Geometry check sheet. Reference: the model listing, model coordinates, mm. A direction names the side the tool comes from. Coordinates: 2 decimals unless noted, no trailing zeros. Loops run counter-clockwise (first coordinate to the right, second up) from the corner with the lowest first, then second, coordinate; pieces in that order, holes last. Notation, with made-up numbers: (45.25, 0.5) -> (62.25, 0.5) arc R15 cw to (62.25, 7.5) -> close; hole circle Ø11 at (57, 48.25). An arc over 180 degrees is marked (long way). Answer as a JSON object with one key per item and string values.
from build123d import *

# Parameters (mm, degrees)
ESQUISSE1_W             = 33.4
ESQUISSE1_H             = 33.4
BOSS_EXTRU_1_DEPTH      = 7
ESQUISSE2_R             = 8.175
ENL_V_MAT_EXTRU_1_DEPTH = 3
ESQUISSE3_W             = 39.4
ESQUISSE3_H             = 39.4
BOSS_EXTRU_2_DEPTH      = 2
BOSS_EXTRU_3_DEPTH      = 10
CONG_1_R                = 2


with BuildPart() as part:
    # Esquisse1 → Boss.-Extru.1 (new body)
    with BuildSketch(Plane.XY):
        Rectangle(ESQUISSE1_W, ESQUISSE1_H)
    extrude(amount=BOSS_EXTRU_1_DEPTH)

    # Esquisse2 → Enlèv. mat.-Extru.1 (cut)
    with BuildSketch(Plane.XY.offset(7)):
        with Locations((0, -2.7)):
            Circle(ESQUISSE2_R)
    extrude(amount=-ENL_V_MAT_EXTRU_1_DEPTH, mode=Mode.SUBTRACT)

    # Esquisse3 → Boss.-Extru.2 (add)
    with BuildSketch(Plane(origin=(0, 0, 0), x_dir=(-1, 0, 0), z_dir=(0, 0, -1))):
        Rectangle(ESQUISSE3_W, ESQUISSE3_H)
    extrude(amount=BOSS_EXTRU_2_DEPTH)

    # Esquisse4 → Boss.-Extru.3 (add)
    with BuildSketch(Plane(origin=(0, 0, -2), x_dir=(-1, 0, 0), z_dir=(0, 0, -1))):
        Polygon((19.7, 19.7), (-19.7, 19.7), (-19.7, -19.7), (-16.7, -19.7), (-16.7, 16.7), (19.7, 16.7), align=None)
    extrude(amount=BOSS_EXTRU_3_DEPTH)

    # Congé1
    cong_1_edges = [part.edges().sort_by_distance(p)[0] for p in [
        (19.7, 19.7, -6),
        (-16.7, 16.7, 3.5),
        (16.7, 16.7, 3.5),
        (16.7, -16.7, 3.5),
        (-16.7, -16.7, 3.5),
    ]]
    fillet(cong_1_edges, radius=CONG_1_R)


solid = part.part
1. Tool access check on faces 1 (the face through (0, -3, 4)), 2 (the face through (-16.1, -16.13, 3.55)), 3 (the face through (0, -16.7, 3)). Record the directions out of +Z, -Z, +X, -X, +Y, -Y that give a thin tool (end or side, any length) a straight path to the whole face; none if there is none.
Evaluation:
{"face 1": "+Z", "face 2": "+Z, -X, -Y", "face 3": "+Z, +X, -X, -Y"}
2. Section check A-A, the plane y = -2.7. Record the boundary of the cut face in (x, z) (3 decimals), then the cut area to 3 significant figures.
Evaluation:
{"outline": "(-19.7, -2) -> (16.7, -2) -> (16.7, -12) -> (19.7, -12) -> (19.7, 0) -> (16.7, 0) -> (16.7, 7) -> (8.175, 7) -> (8.175, 4) -> (-8.175, 4) -> (-8.175, 7) -> (-16.7, 7) -> (-16.7, 0) -> (-19.7, 0) -> close", "area": "294 mm^2"}
3. Thickness scan on probe 1 along Y at (x, z) = (0, 6.1) (3 decimals); probe 2 along X at (y, z) = (2, -7); probe 3 along Z at (x, y) = (3, -2). Record the ranges inside material, lowest first. Write a range as from..to.
Evaluation:
{"probe 1": "y = -16.7..-10.875, 5.475..16.7", "probe 2": "x = 16.7..19.7", "probe 3": "z = -2..4"}
4. Section check D-D, the plane x = -11. Record the boundary of the cut face in (y, z), then the cut area to 3 significant figures.
Evaluation:
{"outline": "(-19.7, -2) -> (16.7, -2) -> (16.7, -12) -> (19.7, -12) -> (19.7, 0) -> (16.7, 0) -> (16.7, 7) -> (-16.7, 7) -> (-16.7, 0) -> (-19.7, 0) -> close", "area": "343 mm^2"}
5. Section check C-C, the plane z = -8.25. Record the boundary of the cut face in (x, y), then the cut area to 3 significant figures.
Evaluation:
{"outline": "(-19.7, 16.7) -> (16.7, 16.7) -> (16.7, -19.7) -> (19.7, -19.7) -> (19.7, 17.7) arc R2 ccw to (17.7, 19.7) -> (-19.7, 19.7) -> close", "area": "227 mm^2"}
6. Section check B-B, the plane x = 0. Record the boundary of the cut face in (y, z) (3 decimals).
Evaluation:
{"outline": "(-19.7, -2) -> (16.7, -2) -> (16.7, -12) -> (19.7, -12) -> (19.7, 0) -> (16.7, 0) -> (16.7, 7) -> (5.475, 7) -> (5.475, 4) -> (-10.875, 4) -> (-10.875, 7) -> (-16.7, 7) -> (-16.7, 0) -> (-19.7, 0) -> close"}
7. Depth check by flat-ended pin: P1, Ø7.5, axis at y = 1, z = 2.5, coming from the +X side; P2, Ø8, axis at x = -1, y = 0, coming from the +Z side; P3, Ø1.5, axis at x = -9.5, z = 4, coming from the +Y side; P4, Ø1, axis at y = 15, z = 1.5, coming from the +X side. Enter the tip coordinate at first touch or a pass-through.
Evaluation:
{"P1": "stops at x = 19.7", "P2": "stops at z = 4", "P3": "stops at y = 16.7", "P4": "stops at x = 16.7"}
